from build123d import *

# Parameters (mm, degrees)
F2_R     = 1
F3_DEPTH = 25


with BuildPart() as f1:
    # F0 (on Front) → F1 (revolve)
    with BuildSketch(Plane.XZ):
        with BuildLine():
            Line((-28, 0), (0, 0))
            Line((0, 0), (0, 2))
            Line((0, 2), (-26.5, 2))
            ThreePointArc((-26.5, 2), (-27.207107, 2.292893), (-27.5, 3))
            Line((-27.5, 3), (-27.5, 5))
            Line((-27.5, 5), (-26.5, 6))
            Line((-26.5, 6), (-27.5, 7))
            Line((-27.5, 7), (-30, 7))
            Line((-30, 7), (-30, 2))
            ThreePointArc((-30, 2), (-29.414214, 0.585786), (-28, 0))
        make_face()
    revolve(axis=Axis((0, 0, 1), (0, 0, 1)))

    # F2 (on face) → F3 (cut)
    with BuildSketch(Plane(origin=(0, 0, 0), x_dir=(1, 0, 0), z_dir=(0, 0, -1))):
        Circle(F2_R)
    extrude(amount=-F3_DEPTH, mode=Mode.SUBTRACT)


solid = f1.part
Input: part model. Units: mm. Frame: model coordinates. Coordinates: 2 decimals unless noted, no trailing zeros. Write each loop counter-clockwise with the first axis right and the second up, starting at its lowest first coordinate (ties: lowest second). Pieces come first, ordered by that corner, then holes. Notation, with made-up numbers: M -38,47.25 L 20,47.25 A9 ccw 20,56.25 Z; hole C 54,68.5 d9. An arc over 180 degrees is marked long. Answer as a JSON object with one key per item and string values. Group by question number.
(1) Contact query for flat-ended pins moving along their axis: P1, Ø4, axis at x = 13, z = 5.5, coming from the -Y side; P2, Ø2, axis at x = 19.5, z = 1.5, coming from the -Y side; P3, Ø3, axis at x = -18, z = 2.5, coming from the +Y side; P4, Ø1.6, axis at x = 0, y = 0, coming from the +Z side. Output: stop coordinate, or through.
(2) Section A-A on x = 0. Output: boundary loops of the cut face in (y, z).
(3) Ray query, line 1 along Y through (x, z) = (0, 3.9); line 2 along Z through (x, y) = (-16, 17.5); line 3 along Y through (x, z) = (-17.5, 3). Return the intervals inside material, ascending. Write a range as [from, to].
(4) Mould query, pull axis Z, two halves, no side actions, for faces 1 (the face through (0, 6, 0)), 2 (the face through (6, 0, 2)), 3 (the face through (0, 1, 1)), 4 (the face through (5.961, 26.846, 4.014)). Classes: pulls with the +Z half, pulls with the -Z half, needs draft (parallel to the pull), parting line crosses it, or undercut.
Result set:
{
 "1": {"P1": "stops at y = -27.91", "P2": "stops at y = -23.57", "P3": "stops at y = 25.05", "P4": "passes through"},
 "2": {"outline": "M -30,2 A2 ccw -28,0 L -1,0 L -1,2 L -26.5,2 A1 cw -27.5,3 L -27.5,5 L -26.5,6 L -27.5,7 L -30,7 Z; M 1,0 L 28,0 A2 ccw 30,2 L 30,7 L 27.5,7 L 26.5,6 L 27.5,5 L 27.5,3 A1 cw 26.5,2 L 1,2 Z"},
 "3": {"line 1": "y = [-30, -27.5], [27.5, 30]", "line 2": "z = [0, 2]", "line 3": "y = [-24.37, -21.21], [21.21, 24.37]"},
 "4": {"face 1": "pulls with the -Z half", "face 2": "pulls with the +Z half", "face 3": "needs draft", "face 4": "undercut"}
}
